Design review of the part built by this model. Coordinates are the model's own, in mm. A direction names the side the tool comes from. Give positions to 0.01 mm unless a question says otherwise; leave off trailing zeros. Write each loop counter-clockwise with the first axis right and the second up, starting at its lowest first coordinate (ties: lowest second). Pieces come first, ordered by that corner, then holes. Notation, with made-up numbers: (36.5, -32.75) -> (53.5, -32.75) arc R25 cw to (53.5, -11.75) -> close; hole circle Ø1 at (-27, -24). An arc over 180 degrees is marked (long way). Put each result on its own line as item: value. Start each with the question number.
from build123d import *

# Parameters (mm, degrees)
SKETCH1_W                 = 10
SKETCH1_H                 = 29.5
SKETCH1_R                 = 2.75
BOSS_EXTRUDE1_DEPTH       = 15.5
SKETCH15_R                = 2.75
CUT_EXTRUDE5_DEPTH        = 10
SKETCH2_W                 = 85
SKETCH2_H                 = 34.5
SKETCH2_R                 = 5.25
BOSS_EXTRUDE2_DEPTH       = 7.5
SKETCH4_W                 = 85
SKETCH4_H                 = 34.5
BOSS_EXTRUDE3_DEPTH       = 10
SKETCH5_W                 = 10
SKETCH5_H                 = 34.5
BOSS_EXTRUDE4_DEPTH       = 60
SKETCH6_R                 = 5
BOSS_EXTRUDE5_DEPTH       = 5
CUT_EXTRUDE2_DEPTH        = 2.5
SKETCH10_W                = 5
SKETCH10_H                = 18.5
CUT_EXTRUDE4_DEPTH        = 10
F_2_5MM_DOWEL_HOLE1_D     = 2.5
F_2_5MM_DOWEL_HOLE1_DEPTH = 10
F_2_5MM_DOWEL_HOLE1_TIP   = 0.751075774
FILLET1_R                 = 2.5
SKETCH14_R                = 5.25
BOSS_EXTRUDE6_DEPTH       = 2.5
FILLET2_R                 = 2.5
SKETCH17_W                = 145
SKETCH17_H                = 12.5
CUT_EXTRUDE7_DEPTH        = 2.5
CHAMFER1_SIZE             = 2.5


# Some blends are built 0.0001 mm under size
with BuildPart() as part:
    # Sketch1 → Boss-Extrude1 (new, symmetric)
    # profile 1 of 8: a face of its own
    with BuildSketch(Plane.XY):
        with Locations((-37.5, -1.25)):
            Rectangle(SKETCH1_W, SKETCH1_H)
        with Locations((-37.5, -8.5)):
            Circle(SKETCH1_R, mode=Mode.SUBTRACT)
        with Locations((-37.5, 8.5)):
            Circle(SKETCH1_R, mode=Mode.SUBTRACT)
    # profile 2 of 8: a face of its own
    with BuildSketch(Plane.XY):
        Polygon((-32.5, -16), (-42.5, -16), (-42.5, -21), (42.5, -21), (42.5, -16), (32.5, -16), align=None)
    # profile 3 of 8: a face of its own
    with BuildSketch(Plane.XY):
        with Locations((37.5, -1.25)):
            Rectangle(SKETCH1_W, SKETCH1_H)
        with Locations((37.5, -8.5)):
            Circle(SKETCH1_R, mode=Mode.SUBTRACT)
        with Locations((37.5, 8.5)):
            Circle(SKETCH1_R, mode=Mode.SUBTRACT)
    # profile 4 of 8: a face of its own
    with BuildSketch(Plane.XY):
        with Locations((-37.5, 8.5)):
            Circle(SKETCH1_R)
    # profile 5 of 8: a face of its own
    with BuildSketch(Plane.XY):
        with Locations((-37.5, -8.5)):
            Circle(SKETCH1_R)
    # profile 6 of 8: a face of its own
    with BuildSketch(Plane.XY):
        with Locations((37.5, 8.5)):
            Circle(SKETCH1_R)
    # profile 7 of 8: a face of its own
    with BuildSketch(Plane.XY):
        with Locations((37.5, -8.5)):
            Circle(SKETCH1_R)
    # profile 8 of 8: a face of its own
    with BuildSketch(Plane.XY):
        Polygon((42.5, -21), (92.5, -21), (92.5, 13.5), (42.5, 13.5), (42.5, -16), align=None)
    extrude(amount=BOSS_EXTRUDE1_DEPTH, both=True)

    # Sketch15 → Cut-Extrude5 (cut)
    with BuildSketch(Plane(origin=(0, 0, -15.5), x_dir=(-1, 0, 0), z_dir=(0, 0, -1))):
        with Locations((-37.5, 8.5)):
            Circle(SKETCH15_R)
        with Locations((-37.5, -8.5)):
            Circle(SKETCH15_R)
        with Locations((37.5, 8.5)):
            Circle(SKETCH15_R)
        with Locations((37.5, -8.5)):
            Circle(SKETCH15_R)
    extrude(amount=-CUT_EXTRUDE5_DEPTH, mode=Mode.SUBTRACT)

    # Sketch2 → Boss-Extrude2 (add)
    with BuildSketch(Plane.XY.offset(15.5)):
        with Locations((0, -3.75)):
            Rectangle(SKETCH2_W, SKETCH2_H)
        with Locations((-19, 0)):
            Circle(SKETCH2_R, mode=Mode.SUBTRACT)
    extrude(amount=BOSS_EXTRUDE2_DEPTH)

    # Sketch4 → Boss-Extrude3 (add)
    with BuildSketch(Plane(origin=(92.5, 0, 0), x_dir=(0, 0, -1), z_dir=(1, 0, 0))):
        with Locations((8.15, -3.75)):
            Rectangle(SKETCH4_W, SKETCH4_H)
    extrude(amount=BOSS_EXTRUDE3_DEPTH)

    # Sketch5 → Boss-Extrude4 (add)
    with BuildSketch(Plane(origin=(102.5, 0, 0), x_dir=(0, 0, -1), z_dir=(1, 0, 0))):
        with Locations((-29.35, -3.75)):
            Rectangle(SKETCH5_W, SKETCH5_H)
        with Locations((45.65, -3.75)):
            Rectangle(SKETCH5_W, SKETCH5_H)
    extrude(amount=BOSS_EXTRUDE4_DEPTH)

    # Sketch6 → Boss-Extrude5 (add)
    with BuildSketch(Plane(origin=(0, 0, 24.35), x_dir=(-1, 0, 0), z_dir=(0, 0, -1))):
        with Locations(Location((-152.5, -3.75, 0), (0, 0, 270))):
            Circle(SKETCH6_R)
    extrude(amount=BOSS_EXTRUDE5_DEPTH)

    # Sketch8 → Cut-Extrude2 (cut)
    with BuildSketch(Plane.XY.offset(-40.65)):
        with BuildLine():
            ThreePointArc((121.500000004, 1.499999993), (116.250000004, -3.750000007), (121.500000004, -9.000000007))
            Line((121.500000004, -9.000000007), (152.500000004, -11.000000007))
            Line((152.500000004, -11.000000007), (162.5, -11.000000007))
            Line((162.5, -11.000000007), (162.5, 3.499999993))
            Line((162.5, 3.499999993), (152.500000004, 3.499999993))
            Line((152.500000004, 3.499999993), (121.500000004, 1.499999993))
        make_face()
    extrude(amount=-CUT_EXTRUDE2_DEPTH, mode=Mode.SUBTRACT)

    # Sketch10 → Cut-Extrude4 (cut)
    with BuildSketch(Plane.ZY.offset(42.5)):
        with Locations((7, 4.25)):
            Rectangle(SKETCH10_W, SKETCH10_H)
    extrude(amount=-CUT_EXTRUDE4_DEPTH, mode=Mode.SUBTRACT)

    # Ø2.5mm Dowel Hole1
    with Locations(Plane(origin=(0, 0, -50.65), x_dir=(-1, 0, 0), z_dir=(0, 0, -1))):
        with Locations((-132.2, -3.75), (-152.5, -3.75)):
            Hole(F_2_5MM_DOWEL_HOLE1_D / 2, depth=F_2_5MM_DOWEL_HOLE1_DEPTH)
            with Locations((0, 0, -(F_2_5MM_DOWEL_HOLE1_DEPTH + F_2_5MM_DOWEL_HOLE1_TIP / 2))):  # 118° drill point
                Cone(0, F_2_5MM_DOWEL_HOLE1_D / 2, F_2_5MM_DOWEL_HOLE1_TIP, mode=Mode.SUBTRACT)

    # Fillet1
    fillet1_edges = [part.edges().sort_by_distance(p)[0] for p in [
        (92.5, -3.75, -15.5),
        (92.5, -3.75, 15.5),
        (42.5, -3.75, 23),
        (0, 13.5, 23),
        (42.5, -3.75, 15.5),
        (92.5, -3.75, -50.65),
        (92.5, -3.75, 34.35),
        (162.5, -3.75, 34.35),
        (162.5, -3.75, -50.65),
    ]]
    fillet(fillet1_edges, radius=FILLET1_R)

    # Sketch14 → Boss-Extrude6 (add)
    with BuildSketch(Plane(origin=(0, 0, 15.5), x_dir=(-1, 0, 0), z_dir=(0, 0, -1))):
        with Locations((19, 0)):
            Circle(SKETCH14_R)
    extrude(amount=-BOSS_EXTRUDE6_DEPTH)

    # Fillet2
    fillet2_edges = [part.edges().sort_by_distance(p)[0] for p in [
        (-37.5, -5, 9.5),
        (-37.5, -5, 4.5),
    ]]
    fillet(fillet2_edges, radius=FILLET2_R - 0.0001)  # a hair under: the kernel refuses the full size
    fillet2_2_edges = [part.edges().sort_by_distance(p)[0] for p in [
        (-37.5, 13.5, 9.5),
        (-37.5, 13.5, 4.5),
    ]]
    fillet(fillet2_2_edges, radius=FILLET2_R)

    # Sketch17 → Cut-Extrude7 (cut)
    with BuildSketch(Plane.XZ.offset(21)):
        with Locations((30, 7)):
            Rectangle(SKETCH17_W, SKETCH17_H)
    extrude(amount=-CUT_EXTRUDE7_DEPTH, mode=Mode.SUBTRACT)

    # Chamfer1
    # the kernel refuses this chamfer: 2.5 mm, written as the material it takes off along each edge
    with BuildSketch(Plane(origin=(108.92920747, -21, 0.75), x_dir=(0, -0.027495876610586317, -0.9996219169112968), z_dir=(-1, 0, 0))) as chamfer1_piece_1_section:
        Polygon((CHAMFER1_SIZE * 0.999621916911, -CHAMFER1_SIZE * 0.0274958766106), (-CHAMFER1_SIZE * 0.0274958766106, -CHAMFER1_SIZE * 0.999621916911), (0, 0), align=None)
    chamfer1_piece_1 = extrude(amount=157.85841494, mode=Mode.PRIVATE)
    chamfer1_piece_1 = split(chamfer1_piece_1, bisect_by=Plane(origin=(30, -18.5, -0.076010386), z_dir=(0, -1, 0)), keep=Keep.TOP, mode=Mode.PRIVATE)
    add(chamfer1_piece_1, mode=Mode.SUBTRACT)
    with BuildSketch(Plane(origin=(-48.92920747, -21, 13.25), x_dir=(0, 0.9996219169112968, -0.027495876610586317), z_dir=(1, 0, 0))) as chamfer1_piece_2_section:
        Polygon((CHAMFER1_SIZE * 0.999621916911, CHAMFER1_SIZE * 0.0274958766106), (-CHAMFER1_SIZE * 0.0274958766106, CHAMFER1_SIZE * 0.999621916911), (0, 0), align=None)
    chamfer1_piece_2 = extrude(amount=157.85841494, mode=Mode.PRIVATE)
    chamfer1_piece_2 = split(chamfer1_piece_2, bisect_by=Plane(origin=(30, -18.5, 14.076010386), z_dir=(0, -1, 0)), keep=Keep.TOP, mode=Mode.PRIVATE)
    add(chamfer1_piece_2, mode=Mode.SUBTRACT)


solid = part.part
Q1. Machinability: for faces 1 (the face through (67, -3, 15.5)), 2 (the face through (40.247, 8.621, -10.57)), 3 (the face through (157.38, -2.67, 21.88)), 4 (the face through (-2, -5, 23)), which of the approach directions +Z, -Z, +X, -X, +Y, -Y give a long, thin tool a straight path to every point of the face, cutting with its end or side? Answer none if there is none.
Q2. Take a section at B-B on x = 65.5. Give the boundary of the cut face in (y, z).
Q3. Take a section at D-D on z = -36. Give the boundary of the cut face in (x, y), then the cut area to 3 significant figures.
Q4. To check wall thickness, follow probe 1 along X at (y, z) = (5, 4); probe 2 along Y at (x, z) = (-37.5, -9.25); probe 3 along X at (y, z) = (0, 19.8). State the ranges of each line that lie inside material, in increasing order. Write a range as from..to.
Q5. Mouldability with a two-part tool opening along X and no side actions: class faces 5 (the face through (-42.5, -4, 3)), 6 (the face through (0, -16, 0)), 7 (the face through (75, 13.5, -2)) as +X half, -X half, draft (parallel to the pull), parting line (faces both ways), or undercut.
Q6. For pin 1 (8 mm diameter, centred on x = -38, y = 7, fed in from -Z); pin 2 (10 mm diameter, centred on x = 42, y = -14.5, fed in from +Z); pin 3 (1.5 mm diameter, centred on y = -3, z = 14, fed in from +X), all flat-tipped, find the tip position at first contact; note any pin that passes through.
Q7. Take a section at A-A on z = -13. Give the boundary of the cut face in (x, y).
Result:
1. face 1: +Z, +Y, -Y
1. face 2: -Z
1. face 3: none
1. face 4: +Z, -X, +Y, -Y
2. outline: (-21, -15.5) -> (13.5, -15.5) -> (13.5, 15.5) -> (-20.75, 15.5) -> (-18.5, 13.25) -> (-18.5, 0.75) -> (-21, -1.75) -> close
3. outline: (92.5, -21) -> (102.5, -21) -> (102.5, 13.5) -> (92.5, 13.5) -> close
3. area: 345 mm^2
4. probe 1: x = -42.5..-32.5, 32.5..102.5
4. probe 2: y = -21..-11.25, -5.75..5.75, 11.25..13.5
4. probe 3: x = -42.5..-24.25, -13.75..42.5, 92.5..102.5, 149.19..155.81
5. face 5: -X half
5. face 6: undercut
5. face 7: draft
6. pin 1: stops at z = -15.5
6. pin 2: stops at z = 23
6. pin 3: stops at x = 102.5
7. outline: (-42.5, -21) -> (102.5, -21) -> (102.5, 13.5) -> (32.5, 13.5) -> (32.5, -16) -> (-32.5, -16) -> (-32.5, 13.5) -> (-42.5, 13.5) -> close; hole circle Ø5.5 at (-37.5, -8.5); hole circle Ø5.5 at (-37.5, 8.5); hole circle Ø5.5 at (37.5, -8.5); hole circle Ø5.5 at (37.5, 8.5)
